Source: CAD feature listing. Evaluate the final solid. Frame: model axes, mm. A direction names the side the tool comes from. Give positions to 0.01 mm unless a question says otherwise; leave off trailing zeros.
from build123d import *

# Parameters (mm, degrees)
F1_DEPTH = 12
F2_R     = 5.5
F3_R     = 1


with BuildPart() as f1:
    # F0 (on Top) → F1 (new body)
    with BuildSketch(Plane.XY):
        with BuildLine():
            ThreePointArc((-48.598922, -33.453621), (0, 59), (48.598922, -33.453621))
            Line((48.598922, -33.453621), (20, -75))
            Line((20, -75), (22.059276, -76.417526))
            Line((22.059276, -76.417526), (50.658199, -34.871147))
            ThreePointArc((50.658199, -34.871147), (0, 61.5), (-50.658199, -34.871147))
            Line((-50.658199, -34.871147), (-22.059276, -76.417526))
            Line((-22.059276, -76.417526), (-20, -75))
            Line((-20, -75), (-48.598922, -33.453621))
        make_face()
    extrude(amount=F1_DEPTH)

    # F2
    f2_edges = [f1.edges().sort_by_distance(p)[0] for p in [
        (-21.029638, -75.708763, 0),
        (-21.029638, -75.708763, 12),
        (21.029638, -75.708763, 12),
        (21.029638, -75.708763, 0),
    ]]
    fillet(f2_edges, radius=F2_R)

    # F3
    f3_edges = [f1.edges().sort_by_distance(p)[0] for p in [
        (-37.918017, -53.379133, 12),
        (-35.85874, -51.961606, 0),
    ]]
    fillet(f3_edges, radius=F3_R)


solid = f1.part
1) First-contact query: pin 1 Ø6 at (y, z) = (-31, 10) entering from -X; pin 2 Ø10 at (x, y) = (-23, -53.5) entering from +Z; pin 3 Ø1 at (y, z) = (10, 10.5) entering from -X; pin 4 Ø5 at (x, z) = (21, 6.5) entering from +Y. Flat tips, straight axial feed; report the tip coordinate or a pass-through.
Checks:
pin 1: stops at x = -54.76
pin 2: passes through
pin 3: stops at x = -60.76
pin 4: stops at y = 58.65
2) Pull-direction query (Y, two-part tool) for faces 1 (the face through (-34.387, -54.1, 5.93)), 2 (the face through (-36.28, -51.87, 0.29)), 3 (the face through (-37.849, -52.95, 0.285)); classes: +Y half, -Y half, draft (parallel to the pull), parting line (faces both ways), or undercut.
Checks:
face 1: undercut
face 2: undercut
face 3: -Y half
3) Ray query, L1, parallel to X at y = 0, z = 3; L2, parallel to Y at x = 0, z = 6.5; L3, parallel to Y at x = -27, z = 8.5. Return the intervals inside material, ascending.
Checks:
L1: x = -61.5 to -59, 59 to 61.5
L2: y = 59 to 61.5
L3: y = -69.24 to -64.83, 52.46 to 55.26
4) Reachability of faces 4 (the face through (36.28, -51.87, 11.71)), 5 (the face through (21.922, -74.419, 10.346)), 6 (the face through (21.922, -74.419, 1.654)) from +Z, -Z, +X, -X, +Y, -Y: full face, straight path, thin tool, end or side. Return the list, or none.
Checks:
face 4: +Z
face 5: +Z, -Y
face 6: -Z, -Y
